Could you check a few things on this model? Use its own coordinates, in mm. Face numbers are marked on the shaded views. A direction names the side the tool comes from. Give positions to 0.01 mm unless a question says otherwise; leave off trailing zeros. Loops run counter-clockwise (first coordinate to the right, second up) from the corner with the lowest first, then second, coordinate; pieces in that order, holes last.
1. Imagine slicing it at D-D (y = -29). List the corners of the cut face in (x, z) for me.
2. For the marked faces 5, 6 and 7, which set-ups out of +Z, -Z, +X, -X, +Y, -Y let a thin tool reach every point of the face, with its end or its side?
3. Imagine slicing it at C-C (z = 50.8). List the corners of the cut face in (x, y) for me, plus the area to 3 significant figures.
4. Imagine slicing it at A-A (x = 12.7). List the corners of the cut face in (y, z) for me, plus the area to 3 significant figures.
5. Thinking about a two-plate mould opening in X: for the marked faces 1, 2, 3 and 4, which applies, +X half, -X half, draft (parallel to the pull), parting line (faces both ways), or undercut?
6. For P1, Ø10, axis at x = 42.5, y = -42, coming from the +Z side; P2, Ø3, axis at x = 53.5, y = -13, coming from the +Z side; P3, Ø4, axis at y = -27.5, z = 35, coming from the +X side; P4, Ø5, axis at y = -40, z = 16, coming from the +X side, each with a flat end and sliding along its axis, tell me the tip position at first contact or that it passes through.
7. Imagine slicing it at B-B (y = -9). List the corners of the cut face in (x, z) for me, plus the area to 3 significant figures.
8. I need wall thicknesses on line 1 along Z through (x, y) = (12.7, -10.5); line 2 along Z through (x, y) = (32, -39.5); line 3 along Y through (x, z) = (22, 51.5). Which ranges of each line are inside material? Lowest first, please.
```python
from build123d import *

# Parameters (mm, degrees)
F0_R     = 6.35
F1_DEPTH = 25.4
F2_DEPTH = 57.15
F4_DEPTH = 50.8


with BuildPart() as f1:
    # F0 (on Front) → F1 (new body)
    with BuildSketch(Plane.XZ):
        Polygon((38.1, 12.7), (38.1, 0), (88.9, 0), (88.9, 19.05), (44.45, 63.5), (-6.35, 63.5), (-6.35, 31.75), (38.1, 31.75), (38.1, 19.05), (50.8, 19.05), (50.8, 12.7), align=None)
        with Locations((12.7, 50.8)):
            Circle(F0_R, mode=Mode.SUBTRACT)
    extrude(amount=F1_DEPTH)

    # F0 (on Front) → F2 (join)
    with BuildSketch(Plane.XZ):
        Polygon((0, 6.35), (0, 0), (38.1, 0), (38.1, 12.7), (50.8, 12.7), (50.8, 19.05), (38.1, 19.05), (38.1, 31.75), (-6.35, 31.75), (-6.35, 6.35), align=None)
    extrude(amount=F2_DEPTH)

    # F3 (on face) → F4 (cut)
    with BuildSketch(Plane(origin=(0, 0, 0), x_dir=(1, 0, 0), z_dir=(0, 0, -1))):
        Polygon((88.9, 0), (88.9, 15.875), (63.5, 0), align=None)
    extrude(amount=-F4_DEPTH, mode=Mode.SUBTRACT)


solid = f1.part
```
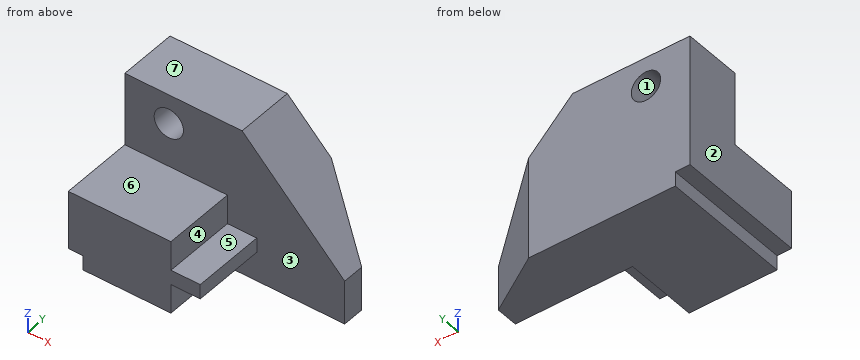
Derived:
1. outline: (-6.35, 6.35) - (0, 6.35) - (0, 0) - (38.1, 0) - (38.1, 12.7) - (50.8, 12.7) - (50.8, 19.05) - (38.1, 19.05) - (38.1, 31.75) - (-6.35, 31.75) - close
2. face 5: +Z, +X, -Y
2. face 6: +Z, +X, -X, -Y
2. face 7: +Z, +X, -X, +Y, -Y
3. outline: (-6.35, -25.4) - (6.35, -25.4) - (6.35, 0) - (-6.35, 0) - close; (19.05, -25.4) - (57.15, -25.4) - (57.15, 0) - (19.05, 0) - close
3. area: 1,290 mm2
4. outline: (-57.15, 0) - (0, 0) - (0, 44.45) - (-25.4, 44.45) - (-25.4, 31.75) - (-57.15, 31.75) - close; (-25.4, 57.15) - (0, 57.15) - (0, 63.5) - (-25.4, 63.5) - close
4. area: 2,300 mm2
5. face 1: undercut
5. face 2: -X half
5. face 3: draft
5. face 4: +X half
6. P1: stops at z = 31.75
6. P2: stops at z = 55.95
6. P3: passes through
6. P4: stops at x = 50.8
7. outline: (-6.35, 6.35) - (0, 6.35) - (0, 0) - (77.9, 0) - (77.9, 30.05) - (44.45, 63.5) - (-6.35, 63.5) - close; hole circle Ø12.7 at (12.7, 50.8)
7. area: 4,620 mm2
8. line 1: z = 0 to 44.45, 57.15 to 63.5
8. line 2: z = 0 to 31.75
8. line 3: y = -25.4 to 0
